Read the model definition and answer for the solid it produces. Units are mm, in the model's axes. Coordinates: 2 decimals unless noted, no trailing zeros. Order: outer loops, then holes, each group sorted by start corner. A loop starts at its lowest first (then second) coordinate and runs counter-clockwise, first axis right, second up. Notation, with made-up numbers: (-5.5, -21.75) -> (29.5, -21.75) arc R24 cw to (29.5, 12.25) -> close; hole circle Ø11 at (9.5, -24). An arc over 180 degrees is marked (long way). Answer in a Markdown table with one row per item.
from build123d import *

# Parameters (mm, degrees)
ESQUISSE2_W = 0.3
ESQUISSE2_H = 4
FENTE_DEPTH = 0.6


with BuildPart() as part:
    # Esquisse1 → Tige (revolve)
    with BuildSketch(Plane.XY, mode=Mode.PRIVATE) as tige_sk:
        with BuildLine():
            Line((0, 0), (1.7, 0))
            Line((1.7, 0), (2, -0.3))
            Line((2, -0.3), (2, -9))
            ThreePointArc((2, -9), (1.118033989, -9.736067977), (0, -10))
            Line((0, -10), (0, 0))
        make_face()
    revolve(tige_sk.sketch.rotate(Axis((0, 0, 0), (0, 1, 0)), 90), axis=Axis((0, 0, 0), (0, 1, 0)))

    # Esquisse2 → Fente (cut)
    with BuildSketch(Plane(origin=(0, 0, 0), x_dir=(1, 0, 0), z_dir=(0, 1, 0))):
        Rectangle(ESQUISSE2_W, ESQUISSE2_H)
    extrude(amount=-FENTE_DEPTH, mode=Mode.SUBTRACT)


solid = part.part
Q1. The part is cut by section B-B (x = 0). Write down the section's boundary in (y, z), then the cut area to 3 significant figures.
Outcome:
| item | result |
|---|---|
| outline | (-9, -2) -> (-0.6, -2) -> (-0.6, 2) -> (-9, 2) arc R2.5 ccw to start |
| area | 36.4 mm² |
Q2. The part is cut by section C-C (y = -2.5). Write down the section's boundary in (x, z), then the cut area to 3 significant figures.
Outcome:
| item | result |
|---|---|
| outline | circle Ø4 at (0, 0) |
| area | 12.6 mm² |
Q3. Given pin 1 (1 mm diameter, centred on x = 1, y = -4, fed in from +Z), flat-ended and moving along its own axis, determine where the tip first touches the part or whether it passes through.
Outcome:
| item | result |
|---|---|
| pin 1 | z = 1.94 |
Q4. The part is cut by section A-A (z = 0). Write down the section's boundary in (x, y).
Outcome:
| item | result |
|---|---|
| outline | (-2, -9) arc R2.5 ccw to (2, -9) -> (2, -0.3) -> (1.7, 0) -> (0.15, 0) -> (0.15, -0.6) -> (-0.15, -0.6) -> (-0.15, 0) -> (-1.7, 0) -> (-2, -0.3) -> close |
Q5. For a pull along X with two mould halves and no side action, classify faces 1 (the face through (-1.82, -0.12, -0.04)), 2 (the face through (1, 0, 0)), 3 (the face through (1.82, -0.12, 0.04)), 4 (the face through (2, -5, 0)) as pulls with the +X half, pulls with the -X half, needs draft (parallel to the pull), parting line crosses it, or undercut.
Outcome:
| item | result |
|---|---|
| face 1 | pulls with the -X half |
| face 2 | needs draft |
| face 3 | pulls with the +X half |
| face 4 | parting line crosses it |
Q6. Consider line 1 (X direction, y = -6.5, z = 1.05); line 2 (X direction, y = -0.5, z = 0.65); line 3 (X direction, y = -5, z = 0.15). Determine where each line is inside the solid, lowest interval first.
Outcome:
| item | result |
|---|---|
| line 1 | -1.7 to 1.7 |
| line 2 | -1.89 to -0.15, 0.15 to 1.89 |
| line 3 | -1.99 to 1.99 |
